from build123d import *

# Parameters (mm, degrees)
SKETCH1_W                = 42.926
SKETCH1_H                = 19.05
BOSS_EXTRUDE1_DEPTH      = 9.525
BOSS_EXTRUDE1_DEPTH_BACK = 9.525
SKETCH2_W                = 23.876
SKETCH2_H                = 9.8806
CUT_EXTRUDE1_DEPTH       = 9.525
CUT_EXTRUDE1_DEPTH_BACK  = 9.525
HOLE1_D                  = 11.32586
HOLE1_DEPTH              = 19.05
HOLE1_CSINK_D            = 12.7
HOLE1_CSINK_ANGLE        = 90


with BuildPart() as part:
    # Sketch1 → Boss-Extrude1 (new body, two sides)
    with BuildSketch(Plane.XY) as boss_extrude1_sk:
        with Locations((11.811, 0)):
            Rectangle(SKETCH1_W, SKETCH1_H)
    extrude(amount=BOSS_EXTRUDE1_DEPTH)
    extrude(boss_extrude1_sk.sketch, amount=-BOSS_EXTRUDE1_DEPTH_BACK)

    # Sketch2 → Cut-Extrude1 (cut, two sides)
    with BuildSketch(Plane(origin=(0, 0, 0), x_dir=(1, 0, 0), z_dir=(0, 1, 0))) as cut_extrude1_sk:
        with Locations((2.286, 0)):
            Rectangle(SKETCH2_W, SKETCH2_H)
    extrude(amount=CUT_EXTRUDE1_DEPTH, mode=Mode.SUBTRACT)
    extrude(cut_extrude1_sk.sketch, amount=-CUT_EXTRUDE1_DEPTH_BACK, mode=Mode.SUBTRACT)

    # Hole1
    with Locations(Plane(origin=(33.274, 0, 0), x_dir=(0, 0, -1), z_dir=(1, 0, 0))):
        with Locations((0, 0)):
            CounterSinkHole(HOLE1_D / 2, HOLE1_CSINK_D / 2, depth=HOLE1_DEPTH, counter_sink_angle=HOLE1_CSINK_ANGLE)

    # Sketch5 → Cut-Revolve1 (revolve, cut)
    with BuildSketch(Plane(origin=(0, 0, 0), x_dir=(0, 0, -1), z_dir=(1, 0, 0))):
        Polygon((-9.525, 0), (-9.525, 5.969), (-8.382, 4.826), (8.382, 4.826), (9.525, 5.969), (9.525, 0), align=None)
    revolve(axis=Axis((0, 0, -9.525), (0, 0, 1)), mode=Mode.SUBTRACT)

    # Sketch6 → Cut-Revolve2 (revolve, cut)
    with BuildSketch(Plane.XY):
        with BuildLine():
            Line((33.274, 0), (33.274, 9.525))
            ThreePointArc((33.274, 9.525), (32.320101294, 14.371793679), (30.734, 19.05))
            Line((30.734, 19.05), (42.799, 19.05))
            Line((42.799, 19.05), (42.799, 0))
            Line((42.799, 0), (33.274, 0))
        make_face()
    revolve(axis=Axis((42.799, 0, 0), (-1, 0, 0)), mode=Mode.SUBTRACT)

    # Sketch7 → Cut-Revolve3 (revolve, cut)
    with BuildSketch(Plane.XY):
        with BuildLine():
            Line((-19.177, 0), (-19.177, 19.05))
            Line((-19.177, 19.05), (-7.112, 19.05))
            ThreePointArc((-7.112, 19.05), (-8.698101294, 14.371793679), (-9.652, 9.525))
            Line((-9.652, 9.525), (-9.652, 0))
            Line((-9.652, 0), (-19.177, 0))
        make_face()
    revolve(axis=Axis((-9.652, 0, 0), (-1, 0, 0)), mode=Mode.SUBTRACT)


solid = part.part
Work out the finished part from the listing and answer in its coordinate system (mm). A direction names the side the tool comes from. Round coordinates to 2 decimals unless told otherwise and drop trailing zeros. Write each loop counter-clockwise with the first axis right and the second up, starting at its lowest first coordinate (ties: lowest second). Pieces come first, ordered by that corner, then holes.
1) Straight lines are drawn through the part: line 1 (Z direction, x = -8, y = -5.5) (3 decimals); line 2 (Z direction, x = 28.5, y = 0) (3 decimals); line 3 (Y direction, x = 0, z = 6.5) (3 decimals). For each, find the intervals that lie inside material, in ascending order.
2) A tool of negligible diameter and unlimited length cuts with its end or side. For faces 4 (the cylindrical face through (2.937, -3.83, 6.637)), 5 (the cylindrical face through (23.277, -5.528, -1.228)), 6 (the flat face through (14.224, -7, 0)), from which of +Z, -Z, +X, -X, +Y, -Y can it reach the whole face along a straight path? Write none if from no direction.
3) Given pin 1 Ø5.5 at (y, z) = (6, 2) entering from -X; pin 2 Ø0.6 at (y, z) = (0.5, 5) entering from +X, each flat-ended and moving along its own axis, determine where each tip first touches the part or whether it passes through.
4) A cutting plane is placed at B-B (x = 0). Give the vertices of the cut face in (y, z) (3 decimals), plus the area to 3 significant figures.
5) The mould has two halves that part along Z. Classify faces 1 (the flat face through (5, 2, -4.94)), 2 (the flat face through (-9.652, 0, -7)), 3 (the flat face through (12, 0, -9.525)): pulls with the +Z half, pulls with the -Z half, needs draft (parallel to the pull), parting line crosses it, or undercut.
6) A cutting plane is placed at D-D (y = 3.5). Give the number of separate pieces and of enclosed holes in the cut face, plus the area to 3 significant figures.
7) A cutting plane is placed at C-C (x = 16.5). Give the vertices of the cut face in (y, z) (3 decimals).
8) A cutting plane is placed at A-A (x = 11). Give the vertices of the cut face in (y, z) (3 decimals).
Completed:
1. line 1: z = -9.525 to -4.94, 4.94 to 9.525
1. line 2: z = -9.525 to -5.663, 5.663 to 9.525
1. line 3: y = -9.525 to -4.826, 4.826 to 9.525
2. face 4: +Z, -Z
2. face 5: +X
2. face 6: -X, +Y, -Y
3. pin 1: stops at x = 14.22
3. pin 2: stops at x = 14.22
4. outline: (-9.525, -9.525) - (-5.969, -9.525) - (-4.826, -8.382) - (-4.826, -4.94) - (-9.525, -4.94) - close; (-9.525, 4.94) - (-4.826, 4.94) - (-4.826, 8.382) - (-5.969, 9.525) - (-9.525, 9.525) - close; (4.826, -8.382) - (5.969, -9.525) - (9.525, -9.525) - (9.525, -4.94) - (4.826, -4.94) - close; (4.826, 4.94) - (9.525, 4.94) - (9.525, 9.525) - (5.969, 9.525) - (4.826, 8.382) - close
4. area: 83.6 mm2
5. face 1: undercut
5. face 2: needs draft
5. face 3: pulls with the -Z half
6. separate pieces: 4
6. enclosed holes: 0
6. area: 347 mm2
7. outline: (-9.525, -9.525) - (9.525, -9.525) - (9.525, 9.525) - (-9.525, 9.525) - close; hole circle Ø11.326 at (0, 0)
8. outline: (-9.525, -9.525) - (9.525, -9.525) - (9.525, -4.94) - (-9.525, -4.94) - close; (-9.525, 4.94) - (9.525, 4.94) - (9.525, 9.525) - (-9.525, 9.525) - close
